Autodesk Inventor part; units mm, degrees
ref_plane "YZ Plane" through (0, 0, 0) normal (1, 0, 0) x (0, 1, 0)
ref_plane "XZ Plane" through (0, 0, 0) normal (0, 1, 0) x (-1, 0, 0)
ref_plane "XY Plane" through (0, 0, 0) normal (0, 0, 1) x (1, 0, 0)
sketch "Sketch1" plane through (0, 0, 0) normal (1, 0, 0) x (0, 1, 0)
  line L0 (-76.2, 88.9) -> (-76.2, 88.9)
  line L1 (-50.8, 127) -> (50.8, 127)
  line L2 (50.8, -127) -> (-50.8, -127)
  line L3 (-76.2, -88.9) -> (-76.2, 88.9)
  arc A0 (88.9, 88.9) -> (50.8, 127) centre (50.8, 88.9) ccw
  line L4 (76.2, 88.9) -> (88.9, 88.9)
  arc A1 (-50.8, 127) -> (-88.9, 88.9) centre (-50.8, 88.9) ccw
  line L5 (-50.8, 88.9) -> (-88.9, 88.9)
  arc A2 (50.8, -127) -> (88.9, -88.9) centre (50.8, -88.9) ccw
  line L6 (76.2, -88.9) -> (88.9, -88.9)
  line L7 (76.2, 88.9) -> (76.2, -88.9)
  arc A3 (-88.9, -88.9) -> (-50.8, -127) centre (-50.8, -88.9) ccw
  line L8 (-76.2, -88.9) -> (-88.9, -88.9)
  point P0 (0, 0)
  point P1 (-76.2, 117.2981)
  point P2 (-76.2, -117.2981)
  dimension "d62" = 254
  dimension "d64" = 76.2
  dimension "d65" = 127
  dimension "d66" = 76.2
  dimension "d72" = 76.2
  dimension "d73" = 25.4
  dimension "d74" = 76.2
  dimension "d76" = 25.4
  dimension "d77" = 76.2
  dimension "d78" = 25.4
extrude "Extrusion1" add sketch "Sketch1" along normal blind 5.08
sketch "Sketch3" plane through (5.08, 0, 0) normal (1, 0, 0) x (0, 0, -1)
  line L0 (88.9, 76.2) -> (-88.9, 76.2)
  line L1 (127, -50.8) -> (127, 50.8)
  line L2 (-88.9, -76.2) -> (88.9, -76.2)
  point P0 (0, 0)
  point P1 (0, -63.5)
  point P2 (0, 63.5)
  point P3 (0, 63.5)
  point P4 (127, 76.2)
  point P5 (127, -76.2)
  point P6 (-127, -76.2)
  dimension "d68" = 12.7
  dimension "d69" = 127
  dimension "d70" = 127
  dimension "d71" = 12.7
sketch "Sketch4" plane through (5.08, 0, 0) normal (1, 0, 0) x (0, 0, -1)
  line L0 (-127, 50.8) -> (-127, -50.8)
  line L1 (-127, 50.8) -> (127, 50.8)
  line L2 (127, 50.8) -> (127, -50.8)
  line L3 (127, -50.8) -> (-127, -50.8)
  line L4 (-127, -50.8) -> (-127, 50.8)
  point P0 (0, 0)
  point P1 (-88.9, 88.9)
  dimension "d79" = 101.6
  dimension "d80" = 38.1
extrude "Extrusion2" add sketch "Sketch4" against normal blind 8.255
sketch "Sketch8" plane through (-3.175, 0, 0) normal (-1, 0, 0) x (0, 0, 1)
  line L0 (-114.3, -44.45) -> (-71.9667, -44.45)
  line L1 (-71.9667, -44.45) -> (-71.9667, -6.35)
  line L2 (-71.9667, -6.35) -> (-114.3, -6.35)
  line L3 (-114.3, -6.35) -> (-114.3, -44.45)
  line L4 (-127, -50.8) -> (127, -50.8)
  line L5 (127, 50.8) -> (-127, 50.8)
  line L6 (-127, 50.8) -> (-127, -50.8)
  line L7 (-127, -50.8) -> (-127, 50.8)
  line L8 (-127, 0) -> (127, 0)
  line L9 (127, 50.8) -> (127, -50.8)
  line L10 (-114.3, 44.45) -> (-71.9667, 44.45)
  line L11 (-71.9667, 44.45) -> (-71.9667, 6.35)
  line L12 (-71.9667, 6.35) -> (-114.3, 6.35)
  line L13 (-114.3, 6.35) -> (-114.3, 44.45)
  line L14 (-15.875, -38.1) -> (15.875, -38.1)
  line L15 (15.875, -38.1) -> (15.875, 38.1)
  line L16 (15.875, 38.1) -> (-15.875, 38.1)
  line L17 (-15.875, 38.1) -> (-15.875, -38.1)
  line L18 (-52.9167, 44.45) -> (-33.8667, 44.45)
  line L19 (-33.8667, 44.45) -> (-33.8667, -44.45)
  line L20 (-33.8667, -44.45) -> (-52.9167, -44.45)
  line L21 (-52.9167, -44.45) -> (-52.9167, 44.45)
  line L22 (-88.9, 76.2) -> (88.9, 76.2)
  line L23 (0, 76.2) -> (0, -76.2)
  line L24 (88.9, -76.2) -> (-88.9, -76.2)
  line L25 (114.3, -44.45) -> (71.9667, -44.45)
  line L26 (71.9667, -44.45) -> (71.9667, -6.35)
  line L27 (71.9667, -6.35) -> (114.3, -6.35)
  line L28 (114.3, -6.35) -> (114.3, -44.45)
  line L29 (114.3, 6.35) -> (114.3, 44.45)
  line L30 (71.9667, 6.35) -> (114.3, 6.35)
  line L31 (114.3, 44.45) -> (71.9667, 44.45)
  line L32 (71.9667, 44.45) -> (71.9667, 6.35)
  line L33 (52.9167, 44.45) -> (33.8667, 44.45)
  line L34 (33.8667, 44.45) -> (33.8667, -44.45)
  line L35 (33.8667, -44.45) -> (52.9167, -44.45)
  line L36 (52.9167, -44.45) -> (52.9167, 44.45)
  point P0 (0, 0)
  dimension "d95" = 6.35
  dimension "d96" = 101.6
  dimension "d97" = 44.45
  dimension "d98" = 12.7
  dimension "d99" = 42.3333
  dimension "d100" = 12.7
  dimension "d101" = 12.7
  dimension "d102" = 31.75
  dimension "d105" = 19.05
  dimension "d106" = 6.35
  dimension "d107" = 6.35
  dimension "d128" = 111.125
  dimension "d129" = 160.8667
extrude "Extrusion5" cut sketch "Sketch8" against normal blind 25.4 contours L3 L2 L1 L0 | L23 L8 L15 L14 | L14 L17 L8 L23 | L21 L18 L19 L8 | L8 L19 L20 L21 | L23 L16 L15 L8 | L8 L17 L16 L23 | L36 L35 L34 L8 | L8 L34 L33 L36 | L10 L11 L12 L13 | L25 L26 L27 L28 | L30 L32 L31 L29
sketch "Sketch10" plane through (0, 0, 0) normal (-1, 0, 0) x (0, 0, 1)
  line L0 (-88.9, 76.2) -> (88.9, 76.2)
  line L1 (0, 76.2) -> (0, -76.2)
  line L2 (88.9, -76.2) -> (-88.9, -76.2)
  line L3 (88.9, 76.2) -> (88.9, 88.9)
  line L4 (127, 50.8) -> (127, -50.8)
  line L5 (127, 0) -> (-127, 0)
  line L6 (-127, 50.8) -> (-127, -50.8)
  point P0 (0, 0)
  point P1 (19.05, 63.5)
  point P2 (69.85, 63.5)
  point P3 (-19.05, 63.5)
  point P4 (-69.85, 63.5)
  point P5 (19.05, -63.5)
  point P6 (69.85, -63.5)
  point P7 (-19.05, -63.5)
  point P8 (-69.85, -63.5)
  dimension "d135" = 12.7
  dimension "d136" = 19.05
  dimension "d137" = 19.05
  dimension "d138" = 12.7
hole "Hole5" at (0, 63.5, 69.85) at (0, 63.5, 19.05) at (0, 63.5, -19.05) at (0, 63.5, -69.85) at (0, -63.5, -69.85) at (0, -63.5, -19.05) at (0, -63.5, 19.05) at (0, -63.5, 69.85) direction (1, 0, 0) diameter 6.35 end through all
sketch "Sketch11" plane through (0, 0, 0) normal (-1, 0, 0) x (0, 0, 1)
  line L0 (50.8, 69.85) -> (38.1, 69.85)
  line L1 (38.1, 69.85) -> (38.1, 57.15)
  line L2 (38.1, 57.15) -> (50.8, 57.15)
  line L3 (50.8, 57.15) -> (50.8, 69.85)
  line L4 (-88.9, 76.2) -> (88.9, 76.2)
  line L5 (127, 50.8) -> (-127, 50.8)
  line L6 (0, 76.2) -> (0, -76.2)
  line L7 (88.9, -76.2) -> (-88.9, -76.2)
  line L8 (0, 69.85) -> (6.35, 69.85)
  line L9 (6.35, 69.85) -> (6.35, 57.15)
  line L10 (6.35, 57.15) -> (0, 57.15)
  circle A0 centre (19.05, 63.5) radius 3.175
  circle A1 centre (69.85, 63.5) radius 3.175
  line L11 (-50.8, 69.85) -> (-38.1, 69.85)
  line L12 (-38.1, 69.85) -> (-38.1, 57.15)
  line L13 (-38.1, 57.15) -> (-50.8, 57.15)
  line L14 (-50.8, 57.15) -> (-50.8, 69.85)
  line L15 (0, 69.85) -> (-6.35, 69.85)
  line L16 (-6.35, 69.85) -> (-6.35, 57.15)
  line L17 (-6.35, 57.15) -> (0, 57.15)
  line L18 (120.0085, -57.15) -> (95.25, -57.15)
  line L19 (95.25, -57.15) -> (95.25, -81.9085)
  arc A2 (95.25, -81.9085) -> (120.0085, -57.15) centre (88.9, -50.8) ccw
  arc A3 (88.9, -88.9) -> (127, -50.8) centre (88.9, -50.8) ccw
  line L20 (-127, -50.8) -> (127, -50.8)
  line L21 (88.9, -88.9) -> (88.9, -76.2)
  line L22 (-120.0085, -57.15) -> (-95.25, -57.15)
  line L23 (-95.25, -57.15) -> (-95.25, -81.9085)
  arc A4 (-120.0085, -57.15) -> (-95.25, -81.9085) centre (-88.9, -50.8) ccw
  line L24 (127, 50.8) -> (127, -50.8)
  line L25 (127, 0) -> (-127, 0)
  line L26 (-127, -50.8) -> (-127, 50.8)
  line L27 (120.0085, 57.15) -> (95.25, 57.15)
  line L28 (95.25, 57.15) -> (95.25, 81.9085)
  arc A5 (120.0085, 57.15) -> (95.25, 81.9085) centre (88.9, 50.8) ccw
  arc A6 (-95.25, 81.9085) -> (-120.0085, 57.15) centre (-88.9, 50.8) ccw
  line L29 (-120.0085, 57.15) -> (-95.25, 57.15)
  line L30 (-95.25, 57.15) -> (-95.25, 81.9085)
  line L31 (50.8, -69.85) -> (38.1, -69.85)
  line L32 (38.1, -69.85) -> (38.1, -57.15)
  line L33 (38.1, -57.15) -> (50.8, -57.15)
  line L34 (50.8, -57.15) -> (50.8, -69.85)
  line L35 (0, -69.85) -> (6.35, -69.85)
  line L36 (6.35, -69.85) -> (6.35, -57.15)
  line L37 (6.35, -57.15) -> (0, -57.15)
  line L38 (-50.8, -57.15) -> (-50.8, -69.85)
  line L39 (-38.1, -57.15) -> (-50.8, -57.15)
  line L40 (-50.8, -69.85) -> (-38.1, -69.85)
  line L41 (-38.1, -69.85) -> (-38.1, -57.15)
  line L42 (-6.35, -69.85) -> (-6.35, -57.15)
  line L43 (-6.35, -57.15) -> (0, -57.15)
  line L44 (0, -69.85) -> (-6.35, -69.85)
  point P0 (0, 0)
  dimension "d146" = 6.35
  dimension "d147" = 6.35
  dimension "d148" = 12.7
  dimension "d149" = 6.35
  dimension "d152" = 19.05
  dimension "d153" = 50.8
  dimension "d154" = 6.35
  dimension "d155" = 6.35
  dimension "d156" = 6.35
  dimension "d159" = 31.75
extrude "Extrusion6" cut sketch "Sketch11" against normal blind 25.4 contours L3 L2 L1 L0 | L17 L16 L15 L6 | L6 L8 L9 L10 | L37 L36 L35 L6 | L6 L44 L42 L43 | L11 L12 L13 L14 | A2 L19 L18 | L22 L23 A4 | L27 L28 A5 | L30 L29 A6 | L31 L32 L33 L34 | L39 L41 L40 L38
properties part number "Frame 2.1" material "ABS Plastic"
The model under review builds one solid part; all positions refer to its coordinate system, in mm. A direction names the side the tool comes from. Round coordinates to 2 decimals unless told otherwise and drop trailing zeros. Order: outer loops, then holes, each group sorted by start corner. A loop starts at its lowest first (then second) coordinate and runs counter-clockwise, first axis right, second up. Notation, with made-up numbers: M 27.5,-31.5 L 57.5,-31.5 A15 ccw 57.5,-17.5 Z; hole C 72.5,-14 d9. An arc over 180 degrees is marked long. Use a Markdown table: item, result.
1) Consider section A-A (z = -42). Write out the cut boundary in (x, y) (3 decimals).
Report:
| item | result |
|---|---|
| outline | M -3.175,-50.8 L 0,-50.8 L 0,-57.15 L 5.08,-57.15 L 5.08,-44.45 L -3.175,-44.45 Z; M -3.175,44.45 L 5.08,44.45 L 5.08,57.15 L 0,57.15 L 0,50.8 L -3.175,50.8 Z; M 0,-76.2 L 5.08,-76.2 L 5.08,-69.85 L 0,-69.85 Z; M 0,69.85 L 5.08,69.85 L 5.08,76.2 L 0,76.2 Z |
2) Consider section C-C (z = 110). Write out the cut boundary in (x, y) (3 decimals).
Report:
| item | result |
|---|---|
| outline | M -3.175,-50.8 L 0,-50.8 L 0,-57.15 L 5.08,-57.15 L 5.08,-44.45 L -3.175,-44.45 Z; M -3.175,-6.35 L 5.08,-6.35 L 5.08,6.35 L -3.175,6.35 Z; M -3.175,44.45 L 5.08,44.45 L 5.08,57.15 L 0,57.15 L 0,50.8 L -3.175,50.8 Z; M 0,-82.524 L 5.08,-82.524 L 5.08,-74.524 L 0,-74.524 Z; M 0,74.524 L 5.08,74.524 L 5.08,82.524 L 0,82.524 Z |
3) Wall thickness on line 1 along Y through (x, z) = (2.6, -69.85) (3 decimals); line 2 along Z through (x, y) = (2.25, 19) (3 decimals); line 3 along Y through (x, z) = (3.5, -3): over which ranges is each line inside the solid? List them lowest first. Write a range as [from, to].
Report:
| item | result |
|---|---|
| line 1 | [-76.2, -66.675], [-60.325, 60.325], [66.675, 76.2] |
| line 2 | [-127, -114.3], [-71.967, -52.917], [-33.867, -15.875], [15.875, 33.867], [52.917, 71.967], [114.3, 127] |
| line 3 | [-76.2, -69.85], [-57.15, -38.1], [38.1, 57.15], [69.85, 76.2] |
4) Consider section B-B (y = -30.5). Write out the cut boundary in (x, z) (3 decimals).
Report:
| item | result |
|---|---|
| outline | M -3.175,-127 L 5.08,-127 L 5.08,-114.3 L -3.175,-114.3 Z; M -3.175,-71.967 L 5.08,-71.967 L 5.08,-52.917 L -3.175,-52.917 Z; M -3.175,-33.867 L 5.08,-33.867 L 5.08,-15.875 L -3.175,-15.875 Z; M -3.175,15.875 L 5.08,15.875 L 5.08,33.867 L -3.175,33.867 Z; M -3.175,52.917 L 5.08,52.917 L 5.08,71.967 L -3.175,71.967 Z; M -3.175,114.3 L 5.08,114.3 L 5.08,127 L -3.175,127 Z |
5) Tool access review of faces 1 (the face through (3, 76.2, 1)), 2 (the face through (3, -64, -38.1)): name each direction out of +Z, -Z, +X, -X, +Y, -Y from which nothing blocks a thin tool from reaching the whole face with its end or side.
Report:
| item | result |
|---|---|
| face 1 | +X, -X, +Y |
| face 2 | +X, -X |
6) Insertion check: pin 1 (2.5 mm diameter, centred on x = 0.5, z = -98.5, fed in from -Y); pin 2 (2.5 mm diameter, centred on x = 0, z = -90.5, fed in from -Y); pin 3 (2.5 mm diameter, centred on x = 4, z = -42.5, fed in from -Y). Each pin has a flat end and moves straight along its axis. Give the tip position at first contact, or say it passes through.
Report:
| item | result |
|---|---|
| pin 1 | y = -87.97 |
| pin 2 | y = -88.9 |
| pin 3 | y = -76.2 |
7) Consider section D-D (x = 1.5). Give the number of separate pieces and of enclosed holes in the cut face, then the cut area to 3 significant figures.
Report:
| item | result |
|---|---|
| separate pieces | 1 |
| enclosed holes | 25 |
| area | 24,200 mm^2 |
8) Draft analysis for pull direction X (two halves, no side actions). For faces 3 (the face through (0, 56.9, 1.8)), 4 (the face through (2.5, 77.44, 116.14)), state which applies: released by +X, released by -X, zero draft, split by the parting line, or undercut.
Report:
| item | result |
|---|---|
| face 3 | released by -X |
| face 4 | zero draft |
